Check sheet for the drawn part. Datum: minimum x, y, z corner. Units: mm. Coordinates: 2 decimals unless noted, no trailing zeros. Loops run counter-clockwise (first coordinate to the right, second up) from the corner with the lowest first, then second, coordinate; pieces in that order, holes last. Notation, with made-up numbers: (9, 48) - (50, 48) arc R21 ccw to (50, 74) - close; hole circle Ø3 at (77, -21.5). An arc over 180 degrees is marked (long way). Write item = value, one per line. Start each with the question number.
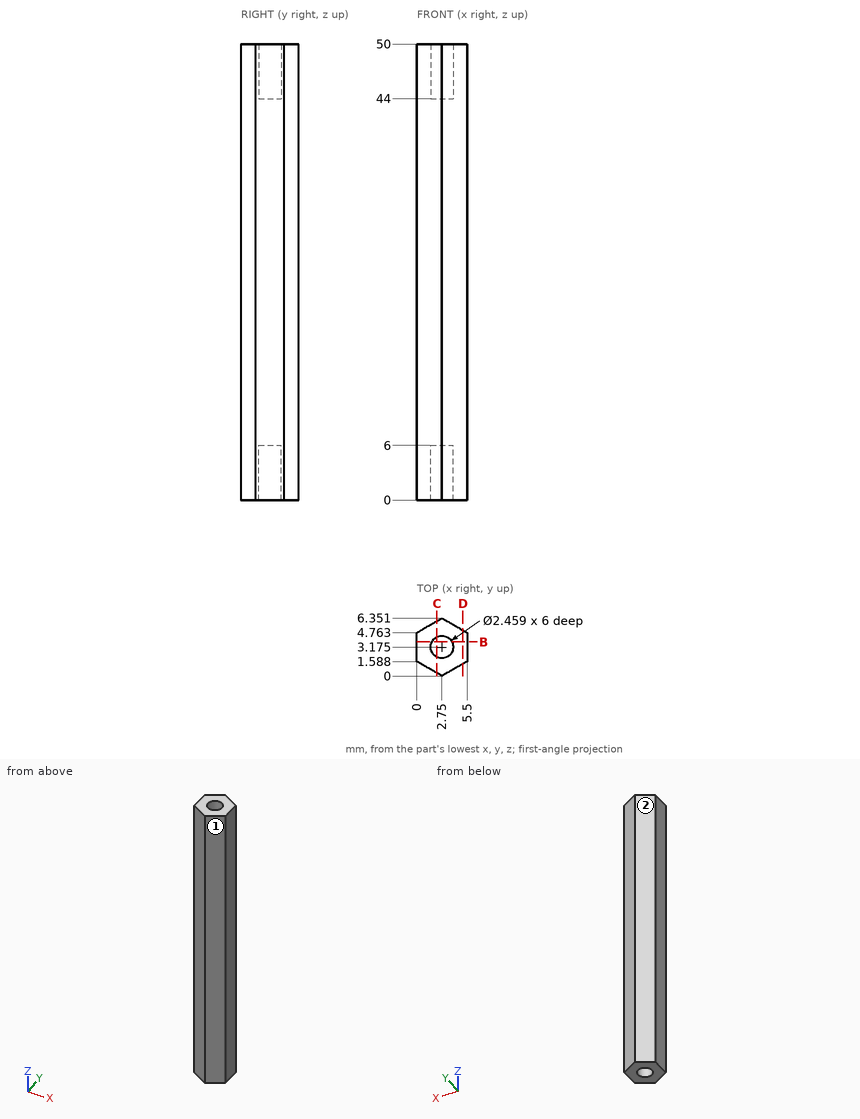
(1) Depth check by flat-ended pin: pin 1 (1.2 mm diameter, centred on x = 3, y = 3.5, fed in from -Z); pin 2 (1 mm diameter, centred on y = 0.5, z = 22, fed in from +X). Enter the tip coordinate at first touch or a pass-through.
(2) Sectioned sample at C-C on x = 2.2. Enter the section's corners in (y, z) (1 decimal).
(3) Scan lines: line 1 (Z direction, x = 3, y = 4); line 2 (X direction, y = 0.75, z = 10); line 3 (X direction, y = 1, z = 16) (1 decimal). Record each from-to range of solid material in increasing order.
(4) Sectioned sample at D-D on x = 5.05. Enter the section's corners in (y, z).
(5) Sectioned sample at B-B on y = 3.75. Enter the section's corners in (x, z).
(6) Draft check along X on the marked faces 1 and 2. Enter one of: pulls with the +X half, pulls with the -X half, needs draft (parallel to the pull), parting line crosses it, or undercut.
Working result:
q1.pin_1 = 6
q1.pin_2 = 4.48
q2.outline = (0.3, 0) - (2.1, 0) - (2.1, 6) - (4.3, 6) - (4.3, 0) - (6, 0) - (6, 50) - (4.3, 50) - (4.3, 44) - (2.1, 44) - (2.1, 50) - (0.3, 50) - close
q3.line_1 = 6 to 44
q3.line_2 = 1.45 to 4.05
q3.line_3 = 1 to 4.5
q4.outline = (1.33, 0) - (5.02, 0) - (5.02, 50) - (1.33, 50) - close
q5.outline = (0, 0) - (1.66, 0) - (1.66, 6) - (3.84, 6) - (3.84, 0) - (5.5, 0) - (5.5, 50) - (3.84, 50) - (3.84, 44) - (1.66, 44) - (1.66, 50) - (0, 50) - close
q6.face_1 = pulls with the +X half
q6.face_2 = pulls with the -X half
